The model under review builds one solid part; all positions refer to its coordinate system, in mm. A direction names the side the tool comes from. Coordinates: 2 decimals unless noted, no trailing zeros. Order: outer loops, then holes, each group sorted by start corner. A loop starts at its lowest first (then second) coordinate and runs counter-clockwise, first axis right, second up.
```python
from build123d import *

# Parameters (mm, degrees)
SKETCH1_W           = 50
SKETCH1_H           = 51
BOSS_EXTRUDE2_DEPTH = 5
BOSS_EXTRUDE3_DEPTH = 5
SKETCH8_W           = 50
SKETCH8_H           = 55
BOSS_EXTRUDE4_DEPTH = 5
SKETCH13_W          = 55
SKETCH13_H          = 51
BOSS_EXTRUDE5_DEPTH = 5
SKETCH14_W          = 50
SKETCH14_H          = 55
BOSS_EXTRUDE6_DEPTH = 5


with BuildPart() as part:
    # Sketch1 → Boss-Extrude2 (new body)
    with BuildSketch(Plane.XY):
        Rectangle(SKETCH1_W, SKETCH1_H)
    extrude(amount=BOSS_EXTRUDE2_DEPTH)

    # Sketch3 → Boss-Extrude3 (add)
    with BuildSketch(Plane(origin=(25, 0, 0), x_dir=(0, 0, -1), z_dir=(1, 0, 0))):
        Polygon((-5, 25.5), (50, 25.5), (50, -25.5), (0, -25.5), (-5, -25.5), align=None)
    extrude(amount=-BOSS_EXTRUDE3_DEPTH)

    # Sketch8 → Boss-Extrude4 (add)
    with BuildSketch(Plane(origin=(0, 25.5, 0), x_dir=(1, 0, 0), z_dir=(0, 1, 0))):
        with Locations((0, 22.5)):
            Rectangle(SKETCH8_W, SKETCH8_H)
    extrude(amount=-BOSS_EXTRUDE4_DEPTH)

    # Sketch13 → Boss-Extrude5 (add)
    with BuildSketch(Plane.ZY.offset(25)):
        with Locations((-22.5, 0)):
            Rectangle(SKETCH13_W, SKETCH13_H)
    extrude(amount=-BOSS_EXTRUDE5_DEPTH)

    # Sketch14 → Boss-Extrude6 (add)
    with BuildSketch(Plane.XZ.offset(25.5)):
        with Locations((0, -22.5)):
            Rectangle(SKETCH14_W, SKETCH14_H)
    extrude(amount=-BOSS_EXTRUDE6_DEPTH)


solid = part.part
```
(1) For pin 1 Ø20 at (x, y) = (7, -2) entering from -Z, flat-tipped, find the tip position at first contact; note if it passes through.
A:
pin 1: stops at z = 0
(2) Wall thickness on probe 1 along X at (y, z) = (12, -36); probe 2 along Y at (x, z) = (4, -8.5); probe 3 along Z at (x, y) = (17, 2.5): over which ranges is each line inside the solid? List them lowest first.
A:
probe 1: x = -25 to -20, 20 to 25
probe 2: y = -25.5 to -20.5, 20.5 to 25.5
probe 3: z = 0 to 5
(3) Draft analysis for pull direction X (two halves, no side actions). For faces 3 (the face through (20, 0, -25)), 4 (the face through (0, -25.5, -23)), 5 (the face through (-25, 0, -23)), state which applies: released by +X, released by -X, zero draft, split by the parting line, or undercut.
A:
face 3: undercut
face 4: zero draft
face 5: released by -X
(4) We need section A-A, the plane z = -45.5. Write out the cut boundary in (x, y), and give its area (3 significant figures).
A:
outline: (-25, -25.5) - (25, -25.5) - (25, 25.5) - (-25, 25.5) - close; hole (-20, -20.5) - (20, -20.5) - (20, 20.5) - (-20, 20.5) - close
area: 910 mm2
(5) Machinability: for faces 1 (the face through (22, 0, -50)), 2 (the face through (0, -20.5, -25)), which of the approach directions +Z, -Z, +X, -X, +Y, -Y give a long, thin tool a straight path to every point of the face, cutting with its end or side? Answer none if there is none.
A:
face 1: -Z, +X, -X, +Y, -Y
face 2: -Z
(6) We need section C-C, the plane x = -10.5. Write out the cut boundary in (y, z), and give its area (3 significant figures).
A:
outline: (-25.5, -50) - (-20.5, -50) - (-20.5, 0) - (20.5, 0) - (20.5, -50) - (25.5, -50) - (25.5, 5) - (-25.5, 5) - close
area: 755 mm2
(7) We need section B-B, the plane y = -12. Write out the cut boundary in (x, z), and give its area (3 significant figures).
A:
outline: (-25, -50) - (-20, -50) - (-20, 0) - (20, 0) - (20, -50) - (25, -50) - (25, 5) - (-25, 5) - close
area: 750 mm2
